from build123d import *

# Parameters (mm, degrees)
CROQUIS1_R              = 3.175
SALIENTE_EXTRUIR1_DEPTH = 2.5
CROQUIS2_R              = 9.921875
CORTAR_EXTRUIR1_DEPTH   = 10


with BuildPart() as part:
    # Croquis1 → Saliente-Extruir1 (new, symmetric)
    with BuildSketch(Plane.XY):
        with BuildLine():
            Line((-123.651340996, 64.638192037), (134.451149425, 37.291264637))
            ThreePointArc((134.451149425, 37.291264637), (168, 0), (134.451149425, -37.291264637))
            Line((134.451149425, -37.291264637), (-123.651340996, -64.638192037))
            ThreePointArc((-123.651340996, -64.638192037), (-195.5, 0), (-123.651340996, 64.638192037))
        make_face()
        with Locations((63.036149834, 3.50684658)):
            Circle(CROQUIS1_R, mode=Mode.SUBTRACT)
        with Locations((33.200158154, 0.374179913)):
            Circle(CROQUIS1_R, mode=Mode.SUBTRACT)
        with Locations((-21.73784786, -5.394103642)):
            Circle(CROQUIS1_R, mode=Mode.SUBTRACT)
        with Locations((8.09814382, -2.261436976)):
            Circle(CROQUIS1_R, mode=Mode.SUBTRACT)
    extrude(amount=SALIENTE_EXTRUIR1_DEPTH, both=True)

    # Croquis2 → Cortar-Extruir1 (cut)
    with BuildSketch(Plane.XY.offset(2.5)):
        with Locations((-130.5, 0)):
            Circle(CROQUIS2_R)
        with Locations((130.5, 0)):
            Circle(CROQUIS2_R)
    extrude(amount=-CORTAR_EXTRUIR1_DEPTH, mode=Mode.SUBTRACT)


solid = part.part
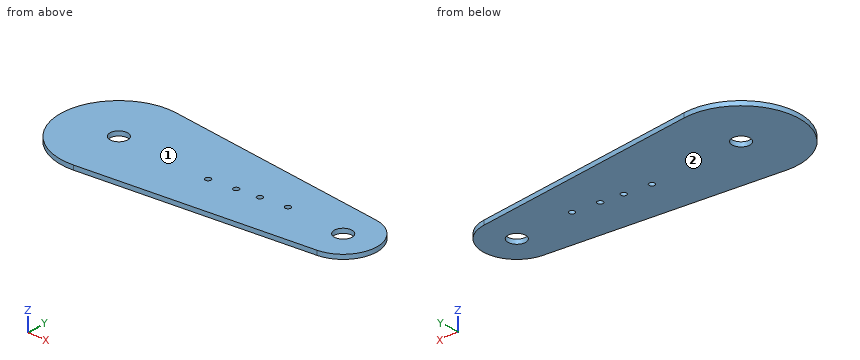
Geometry check sheet. Reference: the model listing, model coordinates, mm. Face numbers are marked on the shaded views. Round coordinates to 2 decimals unless told otherwise and drop trailing zeros. Write each loop counter-clockwise with the first axis right and the second up, starting at its lowest first coordinate (ties: lowest second). Pieces come first, ordered by that corner, then holes.
Item 1: Material ranges on line 1 along Y through (x, z) = (6.5, 0.85); line 2 along X through (y, z) = (33.5, 0); line 3 along Y through (x, z) = (130.5, 0.6), recorded low to high.
Determined:
line 1: y = -50.85 to -5, 0.48 to 50.85
line 2: x = -186.2 to 147.35
line 3: y = -37.71 to -9.92, 9.92 to 37.71
Item 2: Section check B-B (z = 0). Record the boundary of the cut face in (x, y) (3 decimals), plus the area to 3 significant figures.
Determined:
outline: (-123.651, -64.638) - (134.451, -37.291) arc R37.5 ccw to (134.451, 37.291) - (-123.651, 64.638) arc R65 ccw (long way) to start; hole circle Ø19.844 at (-130.5, 0); hole circle Ø6.35 at (-21.738, -5.394); hole circle Ø6.35 at (8.098, -2.261); hole circle Ø6.35 at (33.2, 0.374); hole circle Ø6.35 at (63.036, 3.507); hole circle Ø19.844 at (130.5, 0)
area: 35,000 mm2
Item 3: Mould release check, pull along Z, two halves, no side actions. Record for the marked faces 1 and 2: +Z half, -Z half, draft (parallel to the pull), parting line (faces both ways), or undercut.
Determined:
face 1: +Z half
face 2: -Z half
Item 4: Section check D-D (y = -56). Record the boundary of the cut face in (x, z).
Determined:
outline: (-163.5, -2.5) - (-42.12, -2.5) - (-42.12, 2.5) - (-163.5, 2.5) - close
Item 5: Go/stop test with flat-tipped pins: pin 1 Ø1.5 at (x, z) = (-111.5, -0.5) entering from +Y; pin 2 Ø1.5 at (x, z) = (103, 0) entering from -Y; pin 3 Ø3 at (x, z) = (-58, 2) entering from -Y. Record where each tip stops, or that it passes through.
Determined:
pin 1: stops at y = 63.43
pin 2: stops at y = -40.7
pin 3: stops at y = -57.84
Item 6: Section check C-C (x = 130.5). Record the boundary of the cut face in (y, z), plus the area to 3 significant figures.
Determined:
outline: (-37.71, -2.5) - (-9.92, -2.5) - (-9.92, 2.5) - (-37.71, 2.5) - close; (9.92, -2.5) - (37.71, -2.5) - (37.71, 2.5) - (9.92, 2.5) - close
area: 278 mm2
Item 7: Section check A-A (x = -130.5). Record the boundary of the cut face in (y, z), plus the area to 3 significant figures.
Determined:
outline: (-65, -2.5) - (-9.92, -2.5) - (-9.92, 2.5) - (-65, 2.5) - close; (9.92, -2.5) - (65, -2.5) - (65, 2.5) - (9.92, 2.5) - close
area: 551 mm2
